Here's how the part is built. I have some questions about the finished solid (model axes, mm). A direction names the side the tool comes from. Round coordinates to 2 decimals unless told otherwise and drop trailing zeros. Loops run counter-clockwise (first coordinate to the right, second up) from the corner with the lowest first, then second, coordinate; pieces in that order, holes last. Notation, with made-up numbers: M -26,-13 L 30,-13 A25 ccw 30,4 Z; hole C 66.5,9 d7. An arc over 180 degrees is marked long. Answer as a JSON object with one key per item and string values.
from build123d import *

# Parameters (mm, degrees)
F1_DEPTH = 6
F2_W     = 10
F2_H     = 30
F3_DEPTH = 6
F4_R     = 1.5
F5_DEPTH = 34.001


with BuildPart() as f1:
    # F0 (on Top) → F1 (new body)
    with BuildSketch(Plane.XY):
        Polygon((7, -150), (17, -150), (17, 150), (-17, 150), (-17, -150), (-7, -150), (-7, 10), (-5, 10), (-5, -120), (5, -120), (5, 10), (7, 10), align=None)
    extrude(amount=F1_DEPTH)

    # F2 (on face) → F3 (join)
    with BuildSketch(Plane.XY.offset(6)):
        with Locations((-12, -135)):
            Rectangle(F2_W, F2_H)
        with Locations((12, -135)):
            Rectangle(F2_W, F2_H)
    extrude(amount=F3_DEPTH)

    # F4 (on face) → F5 (cut, through all)
    with BuildSketch(Plane(origin=(-17, 0, 0), x_dir=(0, -1, 0), z_dir=(-1, 0, 0))):
        with Locations((136.304066, 6)):
            Circle(F4_R)
    extrude(amount=-F5_DEPTH, mode=Mode.SUBTRACT)


solid = f1.part
Item 1: I want a section at B-B, the plane z = 2. Please give me the cut outline in (x, y), then the cut area to 3 significant figures.
Resolved:
{"outline": "M -17,-150 L -7,-150 L -7,10 L -5,10 L -5,-120 L 5,-120 L 5,10 L 7,10 L 7,-150 L 17,-150 L 17,150 L -17,150 Z", "area": "9,260 mm²"}
Item 2: Please list where these lines run through material, in increasing order: probe 1 along X at (y, z) = (-21.5, 1.75); probe 2 along X at (y, z) = (-137, 7.75); probe 3 along Z at (x, y) = (1.5, -11). Write a range as from..to.
Resolved:
{"probe 1": "-17..-7, -5..5, 7..17", "probe 2": "-17..-7, 7..17", "probe 3": "0..6"}
Item 3: On a 3-axis mill with a long thin cutter (end or side, diameter ignored), from which of +Z, -Z, +X, -X, +Y, -Y can I reach the whole of each face in a straight line? I mean faces 5 (the face through (0, -120, 3)), 6 (the face through (0, 17, 6)), 7 (the face through (-12, -150, 6)). Say none if no direction works.
Resolved:
{"face 5": "+Z, -Z, -Y", "face 6": "+Z, +X, -X, +Y", "face 7": "+Z, -Z, +X, -X, -Y"}
Item 4: I want a section at C-C, the plane y = 107.5. Please give me the cut outline in (x, z).
Resolved:
{"outline": "M -17,0 L 17,0 L 17,6 L -17,6 Z"}
Item 5: I want a section at D-D, the plane x = 1.5. Please give me the cut outline in (y, z).
Resolved:
{"outline": "M -120,0 L 150,0 L 150,6 L -120,6 Z"}
Item 6: I want a section at A-A, the plane x = 14.5. Please give me the cut outline in (y, z).
Resolved:
{"outline": "M -150,0 L 150,0 L 150,6 L -120,6 L -120,12 L -150,12 Z; hole C -136.3,6 d3"}
Item 7: If we mould it in two halves opening along X, with no side actions, what happens to faces 1 (the face through (7, -87, 5)), 2 (the face through (5, -56, 3)), 3 (the face through (12, -120, 9)), 4 (the face through (-17, -2, 3))? For each: pulls with the +X half, pulls with the -X half, needs draft (parallel to the pull), parting line crosses it, or undercut.
Resolved:
{"face 1": "undercut", "face 2": "undercut", "face 3": "needs draft", "face 4": "pulls with the -X half"}
Item 8: I'm going to push flat-ended pins straight in: pin 1 Ø0.6 at (x, z) = (-5.5, 4) entering from -Y; pin 2 Ø3 at (x, z) = (6, 10) entering from +Y; pin 3 Ø3 at (x, z) = (1.5, 4) entering from -Y; pin 4 Ø3.5 at (y, z) = (-48, 8.5) entering from +X. Where does each tip first touch, or does it pass through?
Resolved:
{"pin 1": "y = 10", "pin 2": "y = -120", "pin 3": "y = -120", "pin 4": "through"}
